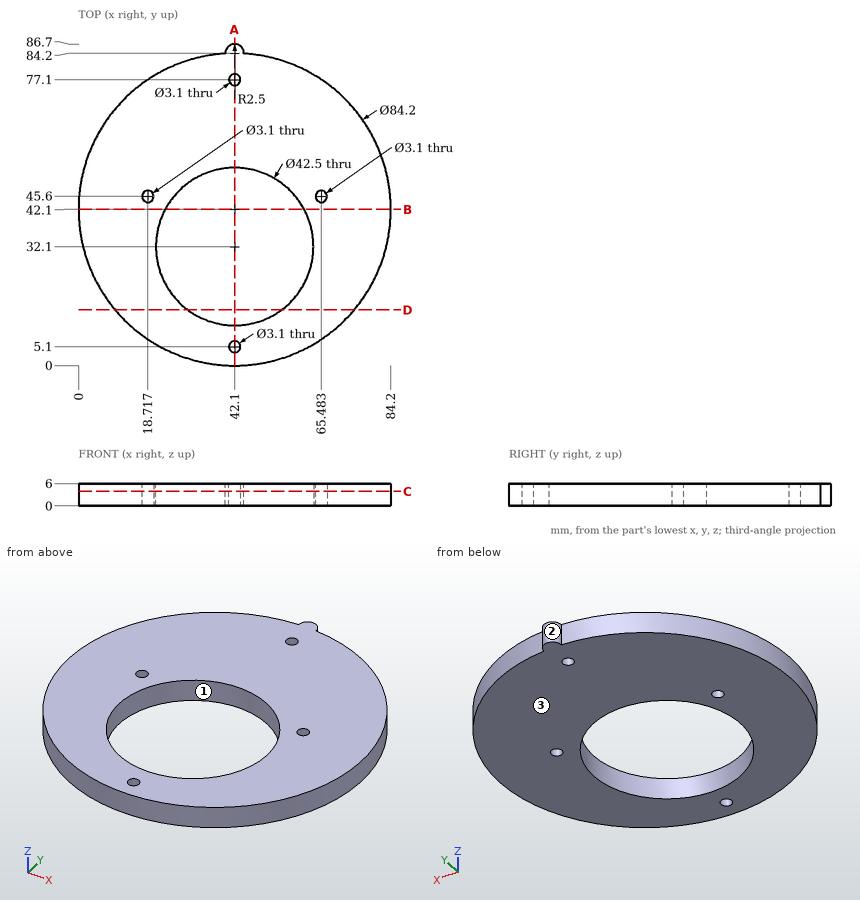
Answer from the drawing. Dimensions are ordinates in mm from the lowest x, y and z of the part. Give positions to 0.01 mm unless a question says otherwise; leave off trailing zeros. Write each loop counter-clockwise with the first axis right and the second up, starting at its lowest first coordinate (ties: lowest second). Pieces come first, ordered by that corner, then holes. Notation, with made-up numbers: (62, 57) - (84, 57) arc R13 ccw to (84, 70) - close; hole circle Ø2 at (36.25, -20.5). An arc over 180 degrees is marked (long way). One line per item, written item: value. Start each with the question number.
1. Find section B-B (y = 42.1). Write down the section's boundary in (x, z).
2. Given pin 1 (12 mm diameter, centred on x = 61.5, y = 39.5, fed in from -Z), flat-ended and moving along its own axis, determine where the tip first touches the part or whether it passes through.
3. Consider probe 1 along Y at (x, z) = (42.1, 2.8); probe 2 along X at (y, z) = (46.5, 2.75) (1 decimal); probe 3 along X at (y, z) = (31, 2.95). Determine where each line is inside the solid, lowest interval first.
4. For a pull along X with two mould halves and no side action, classify the marked faces 1, 2 and 3 as +X half, -X half, draft (parallel to the pull), parting line (faces both ways), or undercut.
5. Find section C-C (z = 3.9). Write down the section's boundary in (x, y), then the cut area to 3 significant figures.
6. Find section D-D (y = 15). Write down the section's boundary in (x, z) (1 decimal).
7. Find section A-A (x = 42.1). Write down the section's boundary in (y, z), then the cut area to 3 significant figures.
Geometry results:
1. outline: (0, 0) - (23.35, 0) - (23.35, 6) - (0, 6) - close; (60.85, 0) - (84.2, 0) - (84.2, 6) - (60.85, 6) - close
2. pin 1: z = 0
3. probe 1: 0 to 3.55, 6.65 to 10.85, 53.35 to 75.55, 78.65 to 86.7
3. probe 2: 0.2 to 17.5, 20 to 26.5, 57.7 to 64.2, 66.7 to 84
3. probe 3: 1.49 to 20.88, 63.32 to 82.71
4. face 1: undercut
4. face 2: parting line
4. face 3: draft
5. outline: (39.6, 84.13) arc R42.1 ccw (long way) to (44.6, 84.13) arc R2.5 ccw (long way) to start; hole circle Ø3.1 at (18.72, 45.6); hole circle Ø42.5 at (42.1, 32.1); hole circle Ø3.1 at (42.1, 5.1); hole circle Ø3.1 at (42.1, 77.1); hole circle Ø3.1 at (65.48, 45.6)
5. area: 4,130 mm2
6. outline: (9.9, 0) - (29.5, 0) - (29.5, 6) - (9.9, 6) - close; (54.7, 0) - (74.3, 0) - (74.3, 6) - (54.7, 6) - close
7. outline: (0, 0) - (3.55, 0) - (3.55, 6) - (0, 6) - close; (6.65, 0) - (10.85, 0) - (10.85, 6) - (6.65, 6) - close; (53.35, 0) - (75.55, 0) - (75.55, 6) - (53.35, 6) - close; (78.65, 0) - (86.7, 0) - (86.7, 6) - (78.65, 6) - close
7. area: 228 mm2
